Part model, mm, in its own coordinate system. A direction names the side the tool comes from. Give positions to 0.01 mm unless a question says otherwise; leave off trailing zeros. Write each loop counter-clockwise with the first axis right and the second up, starting at its lowest first coordinate (ties: lowest second). Pieces come first, ordered by that corner, then holes. Notation, with made-up numbers: M 67.5,32.5 L 121.5,32.5 A29 cw 121.5,55.5 Z; hole C 15.5,80 d9. An arc over 180 degrees is marked long. Use CSV: the item, a comma, the result in double quotes. Start each with the question number.
Item 1: Cut at A-A (x = 30). List the corners of the cut face in (y, z).
Item 2: Which spindle directions (+Z, -Z, +X, -X, +Y, -Y) get a long thin tool onto all of the face, cutting with end or side? Do faces 5 (the flat face through (0, -10, 12)), 6 (the flat face through (22.5, 6, 11)), 7 (the flat face through (0, 12, 2)), 8 (the flat face through (-1.5, 7, 19)), 9 (the cylindrical face through (4.29, -1.93, 14.57)). Say none if no direction does.
Item 3: Mould opens along X. For faces 1 (the flat face through (1.5, 6, 11)), 2 (the flat face through (-0.5, -10.5, 5)), 3 (the flat face through (22.5, 7, 19)), 4 (the flat face through (10.5, 7, 19)) say: released by +X, released by -X, zero draft, split by the parting line, or undercut.
Item 4: Cut at B-B (y = -7.5). List the corners of the cut face in (x, z).
Item 5: Pin check, flat tips, straight feed: pin 1 (2.5 mm diameter, centred on x = 30, y = 0, fed in from -Z); pin 2 (4 mm diameter, centred on y = 4.5, z = 13, fed in from -X); pin 3 (5.5 mm diameter, centred on x = -20, z = 11.5, fed in from -Y); pin 4 (3 mm diameter, centred on x = 22.5, y = 5, fed in from +Z). Stop position of each tip, or through.
Item 6: Drill centre lines: line 1 (X direction, y = 8, z = 19.5); line 2 (X direction, y = 3.5, z = 9.75); line 3 (Y direction, x = -6, z = 14). Where is each one in solid material? Low to high. Write a range as [from, to].
Item 7: Cut at D-D (y = 3.25). Count the separate pieces of the cut face and the enclosed holes in it, then the cut area to 3 significant figures.
Item 8: Cut at C-C (z = 7.5). List the corners of the cut face in (x, y), then the cut area to 3 significant figures.
from build123d import *

# Parameters (mm, degrees)
SKETCH1_W                = 70
SKETCH1_H                = 24
SKETCH1_R                = 1.5
BOSS_EXTRUDE1_DEPTH      = 5
BOSS_EXTRUDE2_DEPTH      = 25.5
BOSS_EXTRUDE2_DEPTH_BACK = 25.5
SKETCH3_R                = 2.321982534
SKETCH3_R_2              = 2.416824645
SKETCH3_W                = 9
SKETCH3_H                = 8
CUT_EXTRUDE1_DEPTH       = 10
BOSS_EXTRUDE3_DEPTH      = 9
BOSS_EXTRUDE4_DEPTH      = 9
BOSS_EXTRUDE5_DEPTH      = 9
BOSS_EXTRUDE6_DEPTH      = 9


with BuildPart() as part:
    # Sketch1 → Boss-Extrude1 (new body)
    with BuildSketch(Plane.XY):
        Rectangle(SKETCH1_W, SKETCH1_H)
        with Locations((-30, 0)):
            Circle(SKETCH1_R, mode=Mode.SUBTRACT)
        with Locations((30, 0)):
            Circle(SKETCH1_R, mode=Mode.SUBTRACT)
    extrude(amount=BOSS_EXTRUDE1_DEPTH)

    # Sketch2 → Boss-Extrude2 (add, two sides: drawn at the far end of the back side and taken through both)
    with BuildSketch(Plane(origin=(0, 0, 0), x_dir=(0, 0, -1), z_dir=(1, 0, 0)).offset(-BOSS_EXTRUDE2_DEPTH_BACK)):
        with BuildLine():
            Line((-5, -10), (-19.5, -10))
            Line((-19.5, -10), (-19.5, 0))
            ThreePointArc((-19.5, 0), (-16.571067812, 7.071067812), (-9.5, 10))
            Line((-9.5, 10), (-5, 10))
            Line((-5, 10), (-5, -10))
        make_face()
    extrude(amount=BOSS_EXTRUDE2_DEPTH + BOSS_EXTRUDE2_DEPTH_BACK)

    # Sketch3 → Cut-Extrude1 (cut)
    with BuildSketch(Plane.XY.offset(19.5)):
        with Locations((6, -3.5)):
            Circle(SKETCH3_R)
        with Locations((18, -3.5)):
            Circle(SKETCH3_R_2)
        with Locations(Location((-18, -3.5, 0), (0, 0, 180))):
            Circle(SKETCH3_R_2)
        with Locations(Location((-6, -3.5, 0), (0, 0, 180))):
            Circle(SKETCH3_R)
        with Locations((6, 4)):
            Rectangle(SKETCH3_W, SKETCH3_H)
        with Locations((18, 4)):
            Rectangle(SKETCH3_W, SKETCH3_H)
        with Locations((-18, 4)):
            Rectangle(SKETCH3_W, SKETCH3_H)
        with Locations((-6, 4)):
            Rectangle(SKETCH3_W, SKETCH3_H)
    extrude(amount=-CUT_EXTRUDE1_DEPTH, mode=Mode.SUBTRACT)

    # Sketch4 → Boss-Extrude3 (add)
    with BuildSketch(Plane.ZY.offset(22.5)):
        with BuildLine():
            Line((9.015316461, 0), (19.5, 0))
            add(Edge.make_bspline(
                [(19.5, 0), (19.395916198, 1.673959857), (19.680366362, 5.037515591), (20.950052063, 8.432343367), (21.831203798, 10.137575266)],
                knots=[0, 0, 0, 0, 0.423484127, 0.846968255, 0.846968255, 0.846968255, 0.846968255], degree=3))
            ThreePointArc((21.831203798, 10.137575266), (21.720999609, 11.224662671), (20.681702642, 11.56195454))
            add(Edge.make_bspline(
                [(20.681702642, 11.56195454), (15.653773695, 10.201988893), (10.35157066, 5.000520578), (9.015316461, 0)],
                knots=[0.123886132, 0.123886132, 0.123886132, 0.123886132, 1, 1, 1, 1], degree=3))
        make_face()
    extrude(amount=-BOSS_EXTRUDE3_DEPTH)

    # Sketch6 → Boss-Extrude4 (add)
    with BuildSketch(Plane(origin=(-10.5, 0, 0), x_dir=(0, 0, -1), z_dir=(1, 0, 0))):
        with BuildLine():
            Line((-9.015316461, 0), (-19.5, 0))
            add(Edge.make_bspline(
                [(-19.5, 0), (-19.395916198, 1.673959857), (-19.680366362, 5.037515591), (-20.950052063, 8.432343367), (-21.831203798, 10.137575266)],
                knots=[0, 0, 0, 0, 0.423484127, 0.846968255, 0.846968255, 0.846968255, 0.846968255], degree=3))
            ThreePointArc((-21.831203798, 10.137575266), (-21.720999609, 11.224662671), (-20.681702642, 11.56195454))
            add(Edge.make_bspline(
                [(-20.681702642, 11.56195454), (-15.653773695, 10.201988893), (-10.35157066, 5.000520578), (-9.015316461, 0)],
                knots=[0.123886132, 0.123886132, 0.123886132, 0.123886132, 1, 1, 1, 1], degree=3))
        make_face()
    extrude(amount=BOSS_EXTRUDE4_DEPTH)

    # Sketch7 → Boss-Extrude5 (add)
    with BuildSketch(Plane(origin=(1.5, 0, 0), x_dir=(0, 0, -1), z_dir=(1, 0, 0))):
        with BuildLine():
            Line((-9.015316461, 0), (-19.5, 0))
            add(Edge.make_bspline(
                [(-19.5, 0), (-19.395916198, 1.673959857), (-19.680366362, 5.037515591), (-20.950052063, 8.432343367), (-21.831203798, 10.137575266)],
                knots=[0, 0, 0, 0, 0.423484127, 0.846968255, 0.846968255, 0.846968255, 0.846968255], degree=3))
            ThreePointArc((-21.831203798, 10.137575266), (-21.720999609, 11.224662671), (-20.681702642, 11.56195454))
            add(Edge.make_bspline(
                [(-20.681702642, 11.56195454), (-15.653773695, 10.201988893), (-10.35157066, 5.000520578), (-9.015316461, 0)],
                knots=[0.123886132, 0.123886132, 0.123886132, 0.123886132, 1, 1, 1, 1], degree=3))
        make_face()
    extrude(amount=BOSS_EXTRUDE5_DEPTH)

    # Sketch8 → Boss-Extrude6 (add)
    with BuildSketch(Plane(origin=(13.5, 0, 0), x_dir=(0, 0, -1), z_dir=(1, 0, 0))):
        with BuildLine():
            Line((-9.015316461, 0), (-19.5, 0))
            add(Edge.make_bspline(
                [(-19.5, 0), (-19.395916198, 1.673959857), (-19.680366362, 5.037515591), (-20.950052063, 8.432343367), (-21.831203798, 10.137575266)],
                knots=[0, 0, 0, 0, 0.423484127, 0.846968255, 0.846968255, 0.846968255, 0.846968255], degree=3))
            ThreePointArc((-21.831203798, 10.137575266), (-21.720999609, 11.224662671), (-20.681702642, 11.56195454))
            add(Edge.make_bspline(
                [(-20.681702642, 11.56195454), (-15.653773695, 10.201988893), (-10.35157066, 5.000520578), (-9.015316461, 0)],
                knots=[0.123886132, 0.123886132, 0.123886132, 0.123886132, 1, 1, 1, 1], degree=3))
        make_face()
    extrude(amount=BOSS_EXTRUDE6_DEPTH)


solid = part.part
Worked answers:
1,outline,"M -12,0 L -1.5,0 L -1.5,5 L -12,5 Z; M 1.5,0 L 12,0 L 12,5 L 1.5,5 Z"
2,face 5,"+Z, +X, -X, -Y"
2,face 6,"none"
2,face 7,"+Z, -Z, +X, -X, +Y"
2,face 8,"+Z, +Y"
2,face 9,"+Z"
3,face 1,"undercut"
3,face 2,"zero draft"
3,face 3,"released by +X"
3,face 4,"undercut"
4,outline,"M -35,0 L 35,0 L 35,5 L 25.5,5 L 25.5,19.5 L -25.5,19.5 L -25.5,5 L -35,5 Z"
5,pin 1,"passes through"
5,pin 2,"stops at x = -25.5"
5,pin 3,"stops at y = -10"
5,pin 4,"stops at z = 20.32"
6,line 1,"x = [-22.5, -13.5], [-10.5, -1.5], [1.5, 10.5], [13.5, 22.5]"
6,line 2,"x = [-25.5, -22.5], [-13.5, -10.5], [-1.5, 1.5], [10.5, 13.5], [22.5, 25.5]"
6,line 3,"y = [-10, -5.82], [-1.18, 7.66], [8, 8.93]"
7,separate pieces,"1"
7,enclosed holes,"4"
7,area,"1,050 mm^2"
8,outline,"M -25.5,-10 L 25.5,-10 L 25.5,10 L -25.5,10 Z"
8,area,"1,020 mm^2"
